```python
from build123d import *

# Parameters (mm, degrees)
SKETCH1_R          = 2.85
EXTRUDE1_DEPTH     = 8
EXTRUDE1_TAPER     = 3
SHELL1_T           = -0.5
SKETCH3_R          = 0.75
EXTRUDE2_DEPTH     = 8
EXTRUDE3_DEPTH     = 4
SKETCH5_R          = 0.398521604
CUT_EXTRUDE1_DEPTH = 10.407178171


with BuildPart() as part:
    # Sketch1 → Extrude1 (new body)
    with BuildSketch(Plane(origin=(0, 0, 0), x_dir=(1, 0, 0), z_dir=(0, 1, 0))):
        Circle(SKETCH1_R)
    extrude(amount=EXTRUDE1_DEPTH, taper=EXTRUDE1_TAPER)

    # Shell1
    shell1_openings = [part.faces().sort_by_distance(p)[0] for p in [
        (0, 0, 0),
    ]]
    offset(amount=SHELL1_T, openings=shell1_openings, kind=Kind.INTERSECTION)

    # Sketch3 → Extrude2 (add)
    with BuildSketch(Plane(origin=(0, 8, 0), x_dir=(-1, 0, 0), z_dir=(0, 1, 0))):
        with Locations(Location((0, 0, 0), (0, 0, 90))):
            Circle(SKETCH3_R)
    extrude(amount=EXTRUDE2_DEPTH)

    # Sketch4 → Extrude3 (add)
    with BuildSketch(Plane(origin=(0, 8, 0), x_dir=(-1, 0, 0), z_dir=(0, 1, 0))):
        with BuildLine():
            Line((0.664541882, 0.323529903), (2.154187801, 0.807545202))
            Line((2.154187801, 0.807545202), (2.2159912, 0.617333899))
            Line((2.2159912, 0.617333899), (0.7269532, 0.133516124))
            ThreePointArc((0.7269532, 0.133516124), (0.702204351, 0.230643797), (0.664541882, 0.323529903))
        make_face()
        with BuildLine():
            Line((-0.1, 0.732316537), (-0.1, 2.3))
            Line((-0.1, 2.3), (0.1, 2.3))
            Line((0.1, 2.3), (0.1, 0.732316537))
            ThreePointArc((0.1, 0.732316537), (0, 0.739112651), (-0.1, 0.732316537))
        make_face()
        with BuildLine():
            Line((0.512399846, -0.532666789), (1.431361279, -1.797508691))
            Line((1.431361279, -1.797508691), (1.26955788, -1.915065741))
            Line((1.26955788, -1.915065741), (0.350828651, -0.650543441))
            ThreePointArc((0.350828651, -0.650543441), (0.435619772, -0.597095407), (0.512399846, -0.532666789))
        make_face()
        with BuildLine():
            Line((-0.350828651, -0.650543441), (-1.26955788, -1.915065741))
            Line((-1.26955788, -1.915065741), (-1.431361279, -1.797508691))
            Line((-1.431361279, -1.797508691), (-0.512399846, -0.532666789))
            ThreePointArc((-0.512399846, -0.532666789), (-0.435619772, -0.597095407), (-0.350828651, -0.650543441))
        make_face()
        with BuildLine():
            Line((-0.7269532, 0.133516124), (-2.2159912, 0.617333899))
            Line((-2.2159912, 0.617333899), (-2.154187801, 0.807545202))
            Line((-2.154187801, 0.807545202), (-0.664541882, 0.323529903))
            ThreePointArc((-0.664541882, 0.323529903), (-0.702204351, 0.230643797), (-0.7269532, 0.133516124))
        make_face()
    extrude(amount=EXTRUDE3_DEPTH)

    # Sketch5 → Cut-Extrude1 (cut, through all)
    with BuildSketch(Plane.XZ.offset(-7.5)):
        with Locations(Location((0, 0, 0), (0, 0, 270))):
            Circle(SKETCH5_R)
    extrude(amount=-CUT_EXTRUDE1_DEPTH, mode=Mode.SUBTRACT)


solid = part.part
```
Source: CAD feature listing. Evaluate the final solid. Frame: model axes, mm. A direction names the side the tool comes from. Give positions to 0.01 mm unless a question says otherwise; leave off trailing zeros. Write each loop counter-clockwise with the first axis right and the second up, starting at its lowest first coordinate (ties: lowest second). Pieces come first, ordered by that corner, then holes.
1. Pull-direction query (X, two-part tool) for faces 1 (the face through (-1.49, 9.97, 0.38)), 2 (the face through (-1.404, 9.972, 0.564)), 3 (the face through (1.466, 9.972, 0.374)), 4 (the face through (1.42, 9.97, 0.57)); classes: +X half, -X half, draft (parallel to the pull), parting line (faces both ways), or undercut.
2. Section query C-C (y = 4.25). Return the cut outline in (x, z).
3. Material intervals for line 1 along X through (y, z) = (9.75, 0); line 2 along X through (y, z) = (6, 0.25); line 3 along X through (y, z) = (8.75, 0.85), sorted ascending.
4. Access query for faces 5 (the face through (0.81, 9.97, -1.28)), 6 (the face through (-0.29, 11.94, 0.69)), 7 (the face through (-0.97, 9.97, -1.16)), 8 (the face through (0.4, 7.5, 0.4)). Directions: +Z, -Z, +X, -X, +Y, -Y. A direction counts if a zero-diameter tool reaches every point of the face in a straight line with its end or side. Return the directions, or none.
5. Section query B-B (y = 14). Return the cut outline in (x, z).
6. First-contact query: pin 1 (1.7 mm diameter, centred on y = 10.5, z = 1, fed in from +X); pin 2 (1.2 mm diameter, centred on x = 1, z = -1.5, fed in from +Y); pin 3 (2 mm diameter, centred on x = 0.5, z = -0.5, fed in from -Y). Flat tips, straight axial feed; report the tip coordinate or a pass-through.
Output values:
1. face 1: -X half
1. face 2: undercut
1. face 3: +X half
1. face 4: undercut
2. outline: circle Ø5.25 at (0, 0); hole circle Ø4.25 at (0, 0)
3. line 1: x = -0.75 to -0.4, 0.4 to 0.75
3. line 2: x = -2.52 to -2.02, 2.02 to 2.52
3. line 3: x = -0.1 to 0.1
4. face 5: -Z, +Y
4. face 6: +Y
4. face 7: -X, +Y
4. face 8: -Y
5. outline: circle Ø1.5 at (0, 0); hole circle Ø0.8 at (0, 0)
6. pin 1: stops at x = 2.22
6. pin 2: stops at y = 12
6. pin 3: stops at y = 7.5
